Geometry check sheet. Reference: drawing and pictorial views, mm from the part's lowest x, y, z. A direction names the side the tool comes from. Coordinates: 2 decimals unless noted, no trailing zeros. Loops run counter-clockwise (first coordinate to the right, second up) from the corner with the lowest first, then second, coordinate; pieces in that order, holes last. Notation, with made-up numbers: (59.5, 19) -> (89.5, 19) arc R23 ccw to (89.5, 35) -> close; hole circle Ø9 at (-36.5, -39.5). An arc over 180 degrees is marked (long way). Answer as a JSON object with one key per item and string values.
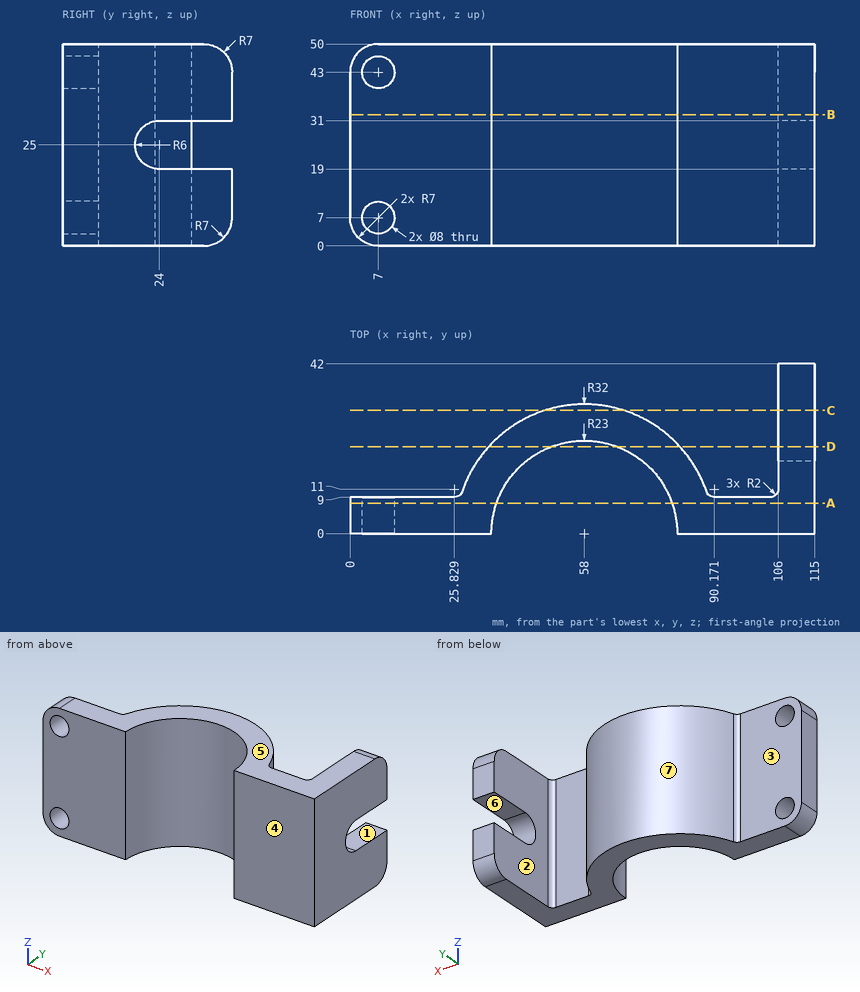
1. Section check C-C, the plane y = 30.5. Record the boundary of the cut face in (x, z).
Evaluation:
{"outline": "(48.32, 0) -> (67.68, 0) -> (67.68, 50) -> (48.32, 50) -> close; (106, 0) -> (115, 0) -> (115, 19) -> (106, 19) -> close; (106, 31) -> (115, 31) -> (115, 50) -> (106, 50) -> close"}
2. Mould release check, pull along Z, two halves, no side actions. Record for the marked faces 5, 6 and 7: released by +Z, released by -Z, zero draft, split by the parting line, or undercut.
Evaluation:
{"face 5": "released by +Z", "face 6": "undercut", "face 7": "zero draft"}
3. Thickness scan on probe 1 along X at (y, z) = (6, 7); probe 2 along X at (y, z) = (2.25, 7); probe 3 along Y at (x, z) = (101.5, 40). Record the ranges inside material, lowest first. Write a range as from..to.
Evaluation:
{"probe 1": "x = 0..3, 11..35.8, 80.2..115", "probe 2": "x = 0..3, 11..35.11, 80.89..115", "probe 3": "y = 0..9"}
4. Section check B-B, the plane z = 32.5. Record the boundary of the cut face in (x, y), then the cut area to 3 significant figures.
Evaluation:
{"outline": "(0, 0) -> (35, 0) arc R23 cw to (81, 0) -> (115, 0) -> (115, 42) -> (106, 42) -> (106, 11) arc R2 cw to (104, 9) -> (90.17, 9) arc R2 cw to (88.28, 10.35) arc R32 ccw to (27.72, 10.35) arc R2 cw to (25.83, 9) -> (0, 9) -> close", "area": "1,540 mm^2"}
5. Tool access check on the marked faces 1, 2, 3 and 4. Record the directions out of +Z, -Z, +X, -X, +Y, -Y that give a thin tool (end or side, any length) a straight path to the whole face; none if there is none.
Evaluation:
{"face 1": "+X, +Y", "face 2": "+Z, -Z, +Y", "face 3": "+Z, -Z, -X, +Y", "face 4": "+Z, -Z, +X, -X, -Y"}
6. Section check D-D, the plane y = 21.5. Record the boundary of the cut face in (x, z) (1 decimal), then the cut area to 4 significant figures.
Evaluation:
{"outline": "(34.3, 0) -> (49.8, 0) -> (49.8, 50) -> (34.3, 50) -> close; (66.2, 0) -> (81.7, 0) -> (81.7, 50) -> (66.2, 50) -> close; (106, 0) -> (115, 0) -> (115, 19.5) -> (106, 19.5) -> close; (106, 30.5) -> (115, 30.5) -> (115, 50) -> (106, 50) -> close", "area": "1,905 mm^2"}
7. Depth check by flat-ended pin: P1, Ø6, axis at y = 36.5, z = 16.5, coming from the -X side; P2, Ø12, axis at x = 49, z = 32, coming from the -Y side (1 decimal); P3, Ø7, axis at x = 99, z = 37, coming from the +Y side; P4, Ø6, axis at x = 32.5, y = 26.5, coming from the +Z side. Enter the tip coordinate at first touch or a pass-through.
Evaluation:
{"P1": "stops at x = 106", "P2": "stops at y = 17.4", "P3": "stops at y = 9", "P4": "passes through"}
8. Section check A-A, the plane y = 7.5. Record the boundary of the cut face in (x, z), then the cut area to 3 significant figures.
Evaluation:
{"outline": "(0, 7) arc R7 ccw to (7, 0) -> (36.26, 0) -> (36.26, 50) -> (7, 50) arc R7 ccw to (0, 43) -> close; (79.74, 0) -> (115, 0) -> (115, 50) -> (79.74, 50) -> close; hole circle Ø8 at (7, 7); hole circle Ø8 at (7, 43)", "area": "3,450 mm^2"}
